Input: part model. Units: mm. Frame: model coordinates. A direction names the side the tool comes from. Give positions to 0.01 mm unless a question says otherwise; leave off trailing zeros. Loops run counter-clockwise (first coordinate to the right, second up) from the corner with the lowest first, then second, coordinate; pieces in that order, holes last. Notation, with made-up numbers: M 31,86 L 68,86 A22 cw 68,97 Z; hole C 32.5,60 d1. An arc over 180 degrees is marked long. Answer as a JSON object with one key per item and string values. Group by question number.
1) Access query for faces 1 (the flat face through (-24.561, 3, -155)), 2 (the flat face through (-28, 3, 35.281)), 3 (the flat face through (165.939, 3, -155)). Directions: +Z, -Z, +X, -X, +Y, -Y. A direction counts if a zero-diameter tool reaches every point of the face in a straight line with its end or side. Return the directions, or none.
2) Section query B-B on z = 91. Return loops of the section in (x, y).
3) Section query A-A on y = 2.75. Return loops of the section in (x, z).
4) First-contact query: P1, Ø1.9, axis at y = 2, z = 79, coming from the -X side; P2, Ø1.9, axis at x = 129, y = 3.5, coming from the -Z side; P3, Ø1.5, axis at y = 3, z = -197, coming from the +X side. Flat tips, straight axial feed; report the tip coordinate or a pass-through.
5) Ray query, L1, parallel to Z at x = 6, y = 2.5; L2, parallel to X at y = 5, z = -130; L3, parallel to Z at x = 84.5, y = 1.5. Return the intervals inside material, ascending.
6) Section query C-C on x = -16. Return loops of the section in (y, z), plus the area to 3 significant figures.
from build123d import *

# Parameters (mm, degrees)
SKETCH1_W           = 203.2
SKETCH1_H           = 304.8
BOSS_EXTRUDE1_DEPTH = 6.35
SKETCH2_W           = 6.35
SKETCH2_H           = 76.2
CUT_EXTRUDE1_DEPTH  = 6.35
SKETCH3_W           = 25.4
SKETCH3_H           = 5.08
BOSS_EXTRUDE3_DEPTH = 6.35
SKETCH5_W           = 44.45
SKETCH5_H           = 6.35
CUT_EXTRUDE2_DEPTH  = 6.35


with BuildPart() as part:
    # Sketch1 → Boss-Extrude1 (new body)
    with BuildSketch(Plane(origin=(0, 0, 0), x_dir=(1, 0, 0), z_dir=(0, 1, 0))):
        with Locations((70.689276808, 40.918703242)):
            Rectangle(SKETCH1_W, SKETCH1_H)
    extrude(amount=BOSS_EXTRUDE1_DEPTH)

    # Sketch2 → Cut-Extrude1 (cut)
    with BuildSketch(Plane(origin=(0, 6.35, 0), x_dir=(1, 0, 0), z_dir=(0, 1, 0))):
        with Locations((-27.735723192, -73.381296758)):
            Rectangle(SKETCH2_W, SKETCH2_H)
        with Locations((-27.735723192, 155.218703242)):
            Rectangle(SKETCH2_W, SKETCH2_H)
        with Locations((169.114276808, 155.218703242)):
            Rectangle(SKETCH2_W, SKETCH2_H)
        with Locations((169.114276808, -73.381296758)):
            Rectangle(SKETCH2_W, SKETCH2_H)
    extrude(amount=-CUT_EXTRUDE1_DEPTH, mode=Mode.SUBTRACT)

    # Sketch3 → Boss-Extrude3 (add)
    with BuildSketch(Plane(origin=(0, 6.35, 0), x_dir=(1, 0, 0), z_dir=(0, 1, 0))):
        with Locations((70.689276808, 195.858703242)):
            Rectangle(SKETCH3_W, SKETCH3_H)
    extrude(amount=-BOSS_EXTRUDE3_DEPTH)

    # Sketch5 → Cut-Extrude2 (cut)
    with BuildSketch(Plane(origin=(0, 6.35, 0), x_dir=(1, 0, 0), z_dir=(0, 1, 0))):
        with Locations((-2.335723192, -108.306296758)):
            Rectangle(SKETCH5_W, SKETCH5_H)
        with Locations((143.714276808, -108.306296758)):
            Rectangle(SKETCH5_W, SKETCH5_H)
    extrude(amount=-CUT_EXTRUDE2_DEPTH, mode=Mode.SUBTRACT)


solid = part.part
Output:
{
 "1": {"face 1": "-Z, -X, +Y, -Y", "face 2": "+Z, -X, +Y, -Y", "face 3": "-Z, +X, +Y, -Y"},
 "2": {"outline": "M -24.56,0 L 165.94,0 L 165.94,6.35 L -24.56,6.35 Z"},
 "3": {"outline": "M -30.91,-117.12 L -24.56,-117.12 L -24.56,-193.32 L 57.99,-193.32 L 57.99,-198.4 L 83.39,-198.4 L 83.39,-193.32 L 165.94,-193.32 L 165.94,-117.12 L 172.29,-117.12 L 172.29,35.28 L 165.94,35.28 L 165.94,105.13 L 121.49,105.13 L 121.49,111.48 L 19.89,111.48 L 19.89,105.13 L -24.56,105.13 L -24.56,35.28 L -30.91,35.28 Z"},
 "4": {"P1": "stops at x = -24.56", "P2": "stops at z = -193.32", "P3": "stops at x = 83.39"},
 "5": {"L1": "z = -193.32 to 105.13", "L2": "x = -24.56 to 165.94", "L3": "z = -193.32 to 111.48"},
 "6": {"outline": "M 0,-193.32 L 6.35,-193.32 L 6.35,105.13 L 0,105.13 Z", "area": "1,900 mm^2"}
}
